from build123d import *

# Parameters (mm, degrees)
SKETCH1_W           = 21
SKETCH1_H           = 12
BOSS_EXTRUDE1_DEPTH = 60
SKETCH2_R           = 2.25
BOSS_EXTRUDE2_DEPTH = 10
SKETCH3_W           = 55
SKETCH3_H           = 18
BOSS_EXTRUDE3_DEPTH = 3
FILLET1_R           = 2


with BuildPart() as part:
    # Sketch1 → Boss-Extrude1 (new body)
    with BuildSketch(Plane.XY):
        Polygon((17.509291985, 21.588576814), (-9.490708015, 21.588576814), (-14.490708015, 21.588576814), (-14.490708015, 18.588576814), (-9.490708015, 18.588576814), (-9.490708015, 6.588576814), (-34.490708015, 6.588576814), (-34.490708015, 18.588576814), (-29.490708015, 18.588576814), (-29.490708015, 21.588576814), (-34.490708015, 21.588576814), (-37.490708015, 21.588576814), (-37.490708015, 3.588576814), (17.509291985, 3.588576814), align=None)
        with Locations((4.009291985, 12.588576814)):
            Rectangle(SKETCH1_W, SKETCH1_H, mode=Mode.SUBTRACT)
    extrude(amount=-BOSS_EXTRUDE1_DEPTH)

    # Sketch2 → Boss-Extrude2 (add)
    # profile 1 of 2: a face of its own
    with BuildSketch(Plane(origin=(-5.490708015, 0, 0), x_dir=(0, 0, -1), z_dir=(1, 0, 0))):
        with BuildLine():
            Line((50, 21.588576814), (40.2, 21.588576814))
            Line((40.2, 21.588576814), (40.2, 33.588576814))
            Line((40.2, 33.588576814), (48, 33.588576814))
            ThreePointArc((48, 33.588576814), (49.414213562, 33.002790376), (50, 31.588576814))
            Line((50, 31.588576814), (50, 21.588576814))
        make_face()
        with Locations(Location((43.5, 27.588576814, 0), (0, 0, 90))):
            Circle(SKETCH2_R, mode=Mode.SUBTRACT)
    # profile 2 of 2: a face of its own
    with BuildSketch(Plane(origin=(-5.490708015, 0, 0), x_dir=(0, 0, -1), z_dir=(1, 0, 0))):
        with BuildLine():
            Line((9.8, 21.588576814), (0, 21.588576814))
            Line((0, 21.588576814), (0, 31.588576814))
            ThreePointArc((0, 31.588576814), (0.585786438, 33.002790376), (2, 33.588576814))
            Line((2, 33.588576814), (9.8, 33.588576814))
            Line((9.8, 33.588576814), (9.8, 21.588576814))
        make_face()
        with Locations(Location((6.5, 27.588576814, 0), (0, 0, 90))):
            Circle(SKETCH2_R, mode=Mode.SUBTRACT)
    extrude(amount=BOSS_EXTRUDE2_DEPTH)

    # Sketch3 → Boss-Extrude3 (add)
    with BuildSketch(Plane(origin=(0, 0, -60), x_dir=(-1, 0, 0), z_dir=(0, 0, -1))):
        with Locations((9.990708015, 12.588576814)):
            Rectangle(SKETCH3_W, SKETCH3_H)
    extrude(amount=BOSS_EXTRUDE3_DEPTH)

    # Fillet1
    fillet1_edges = [part.edges().sort_by_distance(p)[0] for p in [
        (17.509291985, 3.588576814, -31.5),
        (-37.490708015, 3.588576814, -31.5),
        (-37.490708015, 21.588576814, -31.5),
        (17.509291985, 21.588576814, -31.5),
        (4.509291985, 21.588576814, -45.1),
        (-0.490708015, 21.588576814, -50),
        (4.509291985, 21.588576814, -4.9),
        (17.509291985, 12.588576814, -63),
        (-9.990708015, 3.588576814, -63),
        (-37.490708015, 12.588576814, -63),
        (-9.990708015, 21.588576814, -63),
    ]]
    fillet(fillet1_edges, radius=FILLET1_R)


solid = part.part
For this review, take the finished solid that the model builds, in its own axes (mm). A direction names the side the tool comes from. Give positions to 0.01 mm unless a question says otherwise; leave off trailing zeros. Order: outer loops, then holes, each group sorted by start corner. A loop starts at its lowest first (then second) coordinate and runs counter-clockwise, first axis right, second up. Notation, with made-up numbers: (39.25, -17) - (87.25, -17) arc R23 ccw to (87.25, 5) - close; hole circle Ø3 at (53, 66.5). An arc over 180 degrees is marked (long way). Answer as a JSON object with one key per item and string values. Group by question number.
Item 1: Machinability: for faces 1 (the flat face through (4.509, 29, -4)), 2 (the cylindrical face through (-0.561, 32.987, -0.57)), 3 (the flat face through (-32, 18.589, -30)), which of the approach directions +Z, -Z, +X, -X, +Y, -Y give a long, thin tool a straight path to every point of the face, cutting with its end or side? Answer none if there is none.
Item 2: Take a section at B-B on x = -2.5. Give the boundary of the cut face in (y, z), and give its area (3 significant figures).
Item 3: Draft analysis for pull direction Z (two halves, no side actions). For faces 4 (the flat face through (-1, 28, -9.8)), 5 (the flat face through (-14.491, 20, -30)), 6 (the cylindrical face through (-0.561, 33.018, -49.399)), 7 (the flat face through (-8, 14, 0)), state which applies: pulls with the +Z half, pulls with the -Z half, needs draft (parallel to the pull), parting line crosses it, or undercut.
Item 4: Wall thickness on line 1 along X through (y, z) = (17.75, -19); line 2 along Y through (x, z) = (-11, -49); line 3 along Y through (x, z) = (1, -6): over which ranges is each line inside the solid? List them lowest first.
Item 5: Clearance check with flat-ended pins moving along their axes: pin 1 Ø5 at (y, z) = (30.5, -5.5) entering from -X; pin 2 Ø6 at (x, y) = (-2.5, 26) entering from -Z; pin 3 Ø6.5 at (x, y) = (1.5, 27.5) entering from -Z. State where each tip first meets the part, or that it passes through.
Item 6: Take a section at C-C on y = 12. Give the boundary of the cut face in (x, z).
Item 7: Take a section at D-D on x = -30.5. Give the boundary of the cut face in (y, z), and give its area (3 significant figures).
Item 8: Take a section at A-A on z = -6.5. Give the number of separate pieces and of enclosed holes in the cut face, and give its area (3 significant figures).
Reported:
{
 "1": {"face 1": "+Z, -Z, +X, +Y", "face 2": "+Z, +X, -X, +Y", "face 3": "+Z"},
 "2": {"outline": "(3.59, -61) arc R2 ccw to (5.59, -63) - (19.59, -63) arc R2 ccw to (21.59, -61) - (21.59, -52) arc R2 cw to (23.59, -50) - (31.59, -50) arc R2 ccw to (33.59, -48) - (33.59, -40.2) - (21.59, -40.2) - (21.59, -9.8) - (33.59, -9.8) - (33.59, -2) arc R2 ccw to (31.59, 0) - (18.59, 0) - (18.59, -60) - (6.59, -60) - (6.59, 0) - (3.59, 0) - close; hole circle Ø4.5 at (27.59, -43.5); hole circle Ø4.5 at (27.59, -6.5)", "area": "615 mm^2"},
 "3": {"face 4": "undercut", "face 5": "needs draft", "face 6": "pulls with the -Z half", "face 7": "pulls with the +Z half"},
 "4": {"line 1": "-37.49 to -34.49, -9.49 to -6.49, 14.51 to 17.51", "line 2": "3.59 to 6.59, 18.59 to 21.59", "line 3": "3.59 to 6.59, 18.59 to 25.39, 29.78 to 33.59"},
 "5": {"pin 1": "x = -5.49", "pin 2": "z = -50.09", "pin 3": "z = -50"},
 "6": {"outline": "(-37.49, -61) arc R2 ccw to (-35.49, -63) - (15.51, -63) arc R2 ccw to (17.51, -61) - (17.51, 0) - (14.51, 0) - (14.51, -60) - (-6.49, -60) - (-6.49, 0) - (-9.49, 0) - (-9.49, -60) - (-34.49, -60) - (-34.49, 0) - (-37.49, 0) - close"},
 "7": {"outline": "(3.59, -61) arc R2 ccw to (5.59, -63) - (19.59, -63) arc R2 ccw to (21.59, -61) - (21.59, 0) - (18.59, 0) - (18.59, -60) - (6.59, -60) - (6.59, 0) - (3.59, 0) - close", "area": "412 mm^2"},
 "8": {"separate pieces": "2", "enclosed holes": "1", "area": "465 mm^2"}
}
